```python
from build123d import *

# Parameters (mm, degrees)
F0_R     = 2.4257
F1_DEPTH = 3.4544
F2_T     = -0.254
F3_R     = 1.778
F4_DEPTH = 3.81
F5_T     = -0.254


with BuildPart() as f1:
    # F0 (on Front) → F1 (new body)
    with BuildSketch(Plane.XZ):
        Circle(F0_R)
    extrude(amount=F1_DEPTH)

    # F2
    f2_openings = [f1.faces().sort_by_distance(p)[0] for p in [
        (0, -3.4544, 0),
    ]]
    offset(amount=F2_T, openings=f2_openings)

    # F3 (on face) → F4 (join)
    with BuildSketch(Plane(origin=(0, 0, 0), x_dir=(-1, 0, 0), z_dir=(0, 1, 0))):
        Circle(F3_R)
    extrude(amount=F4_DEPTH)

    # F5
    f5_openings = [f1.faces().sort_by_distance(p)[0] for p in [
        (0, 3.81, 0),
    ]]
    offset(amount=F5_T, openings=f5_openings, kind=Kind.INTERSECTION)


solid = f1.part
```
Could you check a few things on this model? Use its own coordinates, in mm. A direction names the side the tool comes from. Round coordinates to 2 decimals unless told otherwise and drop trailing zeros. Write each loop counter-clockwise with the first axis right and the second up, starting at its lowest first coordinate (ties: lowest second). Pieces come first, ordered by that corner, then holes. Notation, with made-up numbers: M 65.25,-32.75 L 77.25,-32.75 A4 ccw 77.25,-26.75 Z; hole C 77.5,82 d7. An arc over 180 degrees is marked long. Answer in a Markdown table with one row per item. Add a question column.
Q1. If I drill on line 1 (Z direction, x = 0.05, y = 2.5); line 2 (Y direction, x = -1.25, z = -0.75), over which ranges is the centre line in solid material (lowest first)? Write a range as from..to.
Q2. Imagine slicing it at D-D (x = 1.65). Please give me the cut outline in (y, z).
Q3. Will these pins go through, and if not, where does the flat tip stop? pin 1 Ø1.5 at (y, z) = (-2, -1.5) entering from -X; pin 2 Ø2.5 at (x, z) = (0, 0) entering from +Y; pin 3 Ø2 at (x, z) = (0.5, 0.5) entering from -Y; pin 4 Ø2.5 at (x, z) = (0.5, 0.5) entering from +Y.
Q4. Imagine slicing it at B-B (z = 0). Please give me the cut outline in (x, y).
Q5. Imagine slicing it at A-A (x = 0). Please give me the cut outline in (y, z).
Q6. Imagine slicing it at C-C (y = -1.5). Please give me the cut outline in (x, z).
Q7. If we mould it in two halves opening along X, with no side actions, what happens to faces 3 (the cylindrical face through (-0.47, -1.83, -2.12)), 4 (the cylindrical face through (2.314, -1.703, 0.729)), 5 (the flat face through (0, 0, 2)), 6 (the cylindrical face through (0.2, 1.88, 1.51))? For each: +X half, -X half, draft (parallel to the pull), parting line (faces both ways), or undercut.
Q8. On a 3-axis mill with a long thin cutter (end or side, diameter ignored), from which of +Z, -Z, +X, -X, +Y, -Y can I reach the whole of each face in a straight line? I mean faces 1 (the cylindrical face through (0.385, 1.878, -1.736)), 2 (the flat face through (0, -0.254, 0)). Say none if no direction works.
Values:
| question | item | result |
|---|---|---|
| 1 | line 1 | -1.78..-1.52, 1.52..1.78 |
| 1 | line 2 | -0.25..0 |
| 2 | outline | M -3.45,-1.78 L 0,-1.78 L 0,-0.66 L 3.81,-0.66 L 3.81,0.66 L 0,0.66 L 0,1.78 L -3.45,1.78 L -3.45,1.41 L -0.25,1.41 L -0.25,-1.41 L -3.45,-1.41 Z |
| 3 | pin 1 | x = -2.31 |
| 3 | pin 2 | y = 0 |
| 3 | pin 3 | y = -0.25 |
| 3 | pin 4 | y = 3.81 |
| 4 | outline | M -2.43,-3.45 L -2.17,-3.45 L -2.17,-0.25 L 2.17,-0.25 L 2.17,-3.45 L 2.43,-3.45 L 2.43,0 L 1.78,0 L 1.78,3.81 L 1.52,3.81 L 1.52,0 L -1.52,0 L -1.52,3.81 L -1.78,3.81 L -1.78,0 L -2.43,0 Z |
| 5 | outline | M -3.45,-2.43 L 0,-2.43 L 0,-1.78 L 3.81,-1.78 L 3.81,-1.52 L 0,-1.52 L 0,1.52 L 3.81,1.52 L 3.81,1.78 L 0,1.78 L 0,2.43 L -3.45,2.43 L -3.45,2.17 L -0.25,2.17 L -0.25,-2.17 L -3.45,-2.17 Z |
| 6 | outline | C 0,0 d4.85; hole C 0,0 d4.34 |
| 7 | face 3 | undercut |
| 7 | face 4 | parting line |
| 7 | face 5 | draft |
| 7 | face 6 | undercut |
| 8 | face 1 | +Y |
| 8 | face 2 | -Y |
